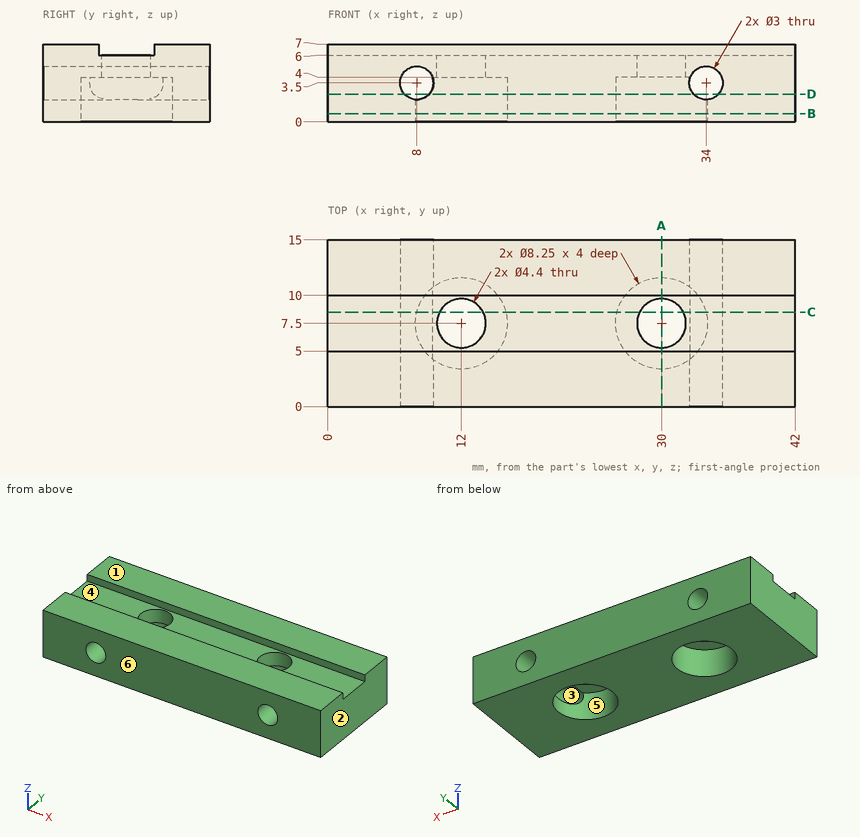
Study the drawing (mm; zero at the part's minimum x, y, z) and answer. A direction names the side the tool comes from. Coordinates: 2 decimals unless noted, no trailing zeros. Write each loop counter-clockwise with the first axis right and the second up, starting at its lowest first coordinate (ties: lowest second). Pieces come first, ordered by that corner, then holes. Notation, with made-up numbers: (36.25, -6.75) - (59.25, -6.75) arc R14 ccw to (59.25, 8.25) - close; hole circle Ø1 at (-9, 7). An arc over 180 degrees is marked (long way). Answer as a JSON object with one key per item and string values. Group by question number.
1. A cutting plane is placed at D-D (z = 2.5). Determine the outline of the cut face in (x, y) (3 decimals).
2. Each of these flat-tipped pins is pushed along its axis until it touches: P1, Ø6.5, axis at x = 30, y = 7.5, coming from the -Z side; P2, Ø1.5, axis at x = 26, y = 6.5, coming from the +Z side. Where does it stop, or does it pass through?
3. A cutting plane is placed at B-B (z = 0.75). Determine the outline of the cut face in (x, y) (3 decimals).
4. A cutting plane is placed at C-C (y = 8.5). Determine the outline of the cut face in (x, z).
5. Consider L1, parallel to Z at x = 34, y = 5.75; L2, parallel to Y at x = 30, z = 4.6; L3, parallel to Y at x = 12, z = 1.55 (3 decimals). Determine where each line is inside the solid, lowest interval first. Write a range as [from, to].
6. Which of the six approach directions +Z, -Z, +X, -X, +Y, -Y give full straight-line access (tool end or side, diameter ignored) to the marked faces 4, 5 and 6?
7. The mould has two halves that part along Z. Classify the marked faces 1, 2 and 3: +Z half, -Z half, draft (parallel to the pull), parting line (faces both ways), or undercut.
8. A cutting plane is placed at A-A (x = 30). Determine the outline of the cut face in (y, z) (3 decimals), plus the area to 3 significant figures.
Worked out:
{
 "1": {"outline": "(0, 0) - (6.882, 0) - (6.882, 15) - (0, 15) - close; (9.118, 0) - (32.882, 0) - (32.882, 4.549) arc R4.125 cw (long way) to (32.882, 10.451) - (32.882, 15) - (9.118, 15) - (9.118, 10.451) arc R4.125 cw (long way) to (9.118, 4.549) - close; (35.118, 0) - (42, 0) - (42, 15) - (35.118, 15) - close"},
 "2": {"P1": "stops at z = 4", "P2": "stops at z = 6"},
 "3": {"outline": "(0, 0) - (42, 0) - (42, 15) - (0, 15) - close; hole circle Ø8.25 at (12, 7.5); hole circle Ø8.25 at (30, 7.5)"},
 "4": {"outline": "(0, 0) - (8, 0) - (8, 2) arc R1.5 cw (long way) to (9.41, 4) - (10.04, 4) - (10.04, 6) - (0, 6) - close; (13.96, 4) - (16, 4) - (16, 0) - (26, 0) - (26, 4) - (28.04, 4) - (28.04, 6) - (13.96, 6) - close; (31.96, 4) - (32.59, 4) arc R1.5 cw (long way) to (34, 2) - (34, 0) - (42, 0) - (42, 6) - (31.96, 6) - close"},
 "5": {"L1": "z = [0, 2], [5, 6]", "L2": "y = [0, 5.3], [9.7, 15]", "L3": "y = [0, 3.375], [11.625, 15]"},
 "6": {"face 4": "+Z, +X, -X", "face 5": "-Z", "face 6": "+Z, -Z, +X, -X, -Y"},
 "7": {"face 1": "+Z half", "face 2": "draft", "face 3": "undercut"},
 "8": {"outline": "(0, 0) - (3.375, 0) - (3.375, 4) - (5.3, 4) - (5.3, 6) - (5, 6) - (5, 7) - (0, 7) - close; (9.7, 4) - (11.625, 4) - (11.625, 0) - (15, 0) - (15, 7) - (10, 7) - (10, 6) - (9.7, 6) - close", "area": "58.2 mm²"}
}
